Input: part model. Units: mm. Frame: model coordinates. Face numbers are marked on the shaded views. A direction names the side the tool comes from. Round coordinates to 2 decimals unless told otherwise and drop trailing zeros. Write each loop counter-clockwise with the first axis right and the second up, starting at its lowest first coordinate (ties: lowest second). Pieces come first, ordered by that corner, then holes. Notation, with made-up numbers: (28, 19) -> (73, 19) arc R18 cw to (73, 44) -> close; hole circle Ø2 at (65.25, 18). An arc over 180 degrees is marked (long way). Write item = value, one per line.
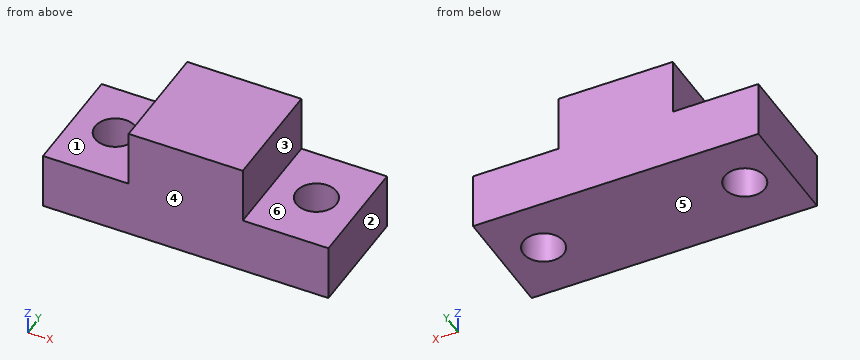
```python
from build123d import *

# Parameters (mm, degrees)
F1_DEPTH = 25.4
F2_R     = 4.468901
F3_DEPTH = 25.4


with BuildPart() as f1:
    # F0 (on Front) → F1 (new body)
    with BuildSketch(Plane.XZ):
        Polygon((0, -25.4), (0, 0), (-12.7, 0), (-12.7, -12.7), (-31.75, -12.7), (-31.75, -25.4), align=None)
    extrude(amount=F1_DEPTH)

    # F2 (on face) → F3 (cut)
    with BuildSketch(Plane.XY.offset(-12.7)):
        with Locations((-22.377703, -12.341406)):
            Circle(F2_R)
    extrude(amount=-F3_DEPTH, mode=Mode.SUBTRACT)

    # F4: F1 across plane


with BuildPart() as f1_1:
    add(f1.part)
    add(f1.part.mirror(Plane.YZ))


solid = f1_1.part
```
1) Access query for the marked faces 1, 2 and 3. Directions: +Z, -Z, +X, -X, +Y, -Y. A direction counts if a zero-diameter tool reaches every point of the face in a straight line with its end or side. Return the directions, or none.
Solutions:
face_1 = +Z, -X, +Y, -Y
face_2 = +Z, -Z, +X, +Y, -Y
face_3 = +Z, +X, +Y, -Y
2) Line query: L1, parallel to X at y = -8.75, z = -9.5; L2, parallel to Z at x = -15.5, y = -24; L3, parallel to X at y = -14.25, z = -15.5. Output: solid intervals per line, ascending. Write a range as from..to.
Solutions:
L1 = -12.7..12.7
L2 = -25.4..-12.7
L3 = -31.75..-26.42, -18.34..18.34, 26.42..31.75
3) Cut plane D-D (y = -23). Return the cut outline in (x, z), and give its area (3 significant figures).
Solutions:
outline = (-31.75, -25.4) -> (31.75, -25.4) -> (31.75, -12.7) -> (12.7, -12.7) -> (12.7, 0) -> (-12.7, 0) -> (-12.7, -12.7) -> (-31.75, -12.7) -> close
area = 1,130 mm^2
4) Cut plane C-C (z = -15.5). Return the cut outline in (x, y).
Solutions:
outline = (-31.75, -25.4) -> (31.75, -25.4) -> (31.75, 0) -> (-31.75, 0) -> close; hole circle Ø8.94 at (-22.38, -12.34); hole circle Ø8.94 at (22.38, -12.34)
5) Cut plane A-A (y = -13). Return the cut outline in (x, z), and give its area (3 significant figures).
Solutions:
outline = (-31.75, -25.4) -> (-26.8, -25.4) -> (-26.8, -12.7) -> (-31.75, -12.7) -> close; (-17.96, -25.4) -> (17.96, -25.4) -> (17.96, -12.7) -> (12.7, -12.7) -> (12.7, 0) -> (-12.7, 0) -> (-12.7, -12.7) -> (-17.96, -12.7) -> close; (26.8, -25.4) -> (31.75, -25.4) -> (31.75, -12.7) -> (26.8, -12.7) -> close
area = 904 mm^2
6) Cut plane B-B (x = -24.5). Return the cut outline in (y, z), and give its area (3 significant figures).
Solutions:
outline = (-25.4, -25.4) -> (-16.27, -25.4) -> (-16.27, -12.7) -> (-25.4, -12.7) -> close; (-8.41, -25.4) -> (0, -25.4) -> (0, -12.7) -> (-8.41, -12.7) -> close
area = 223 mm^2
7) First-contact query: P1, Ø4, axis at y = -16.5, z = -7, coming from the -X side; P2, Ø7, axis at x = -22.38, y = -12.34, coming from the -Z side; P3, Ø9.5, axis at x = 21.5, y = -9, coming from the +Z side; P4, Ø6.5, axis at y = -9.5, z = -8.5, coming from the +X side. Flat tips, straight axial feed; report the tip coordinate or a pass-through.
Solutions:
P1 = -12.7
P2 = through
P3 = -12.7
P4 = 12.7
8) Draft query along Z for the marked faces 4, 5 and 6. Return one class per face: +Z half, -Z half, draft (parallel to the pull), parting line (faces both ways), or undercut.
Solutions:
face_4 = draft
face_5 = -Z half
face_6 = +Z half
